Here's how the part is built. I have some questions about the finished solid (model axes, mm). A direction names the side the tool comes from. Coordinates: 2 decimals unless noted, no trailing zeros. Write each loop counter-clockwise with the first axis right and the second up, starting at its lowest first coordinate (ties: lowest second). Pieces come first, ordered by that corner, then holes. Notation, with made-up numbers: (-2.75, 52) -> (26.25, 52) arc R16 cw to (26.25, 76) -> close; hole circle Ø4 at (70.25, 6). An arc over 180 degrees is marked (long way). Put each result on its own line as item: value. Start each with the question number.
Item 1: For pin 1 (2 mm diameter, centred on x = 0, y = 16, fed in from +Z); pin 2 (3 mm diameter, centred on x = -0.5, y = 1, fed in from -Z); pin 3 (1.3 mm diameter, centred on y = -18, z = 5.5, fed in from -X); pin 4 (3 mm diameter, centred on x = -0.5, y = 8, fed in from +Z), each with a flat end and sliding along its axis, tell me the tip position at first contact or that it passes through.
Item 2: I need wall thicknesses on line 1 (Y direction, x = -2.25, z = 6.5); line 2 (Z direction, x = -3.25, y = -4.5); line 3 (Z direction, x = 1.75, y = -3). Which ranges of each line are inside material? Lowest first, please. Write a range as [from, to].
Item 3: I want a section at B-B, the plane x = -1. List the corners of the cut face in (y, z) for me.
Item 4: I want a section at A-A, the plane z = 4.25. List the corners of the cut face in (x, y) for me.
Item 5: I want a section at C-C, the plane y = 16. List the corners of the cut face in (x, z) for me, then the cut area to 3 significant figures.
Item 6: On a 3-axis mill with a long thin cutter (end or side, diameter ignored), from which of +Z, -Z, +X, -X, +Y, -Y can I reach the whole of each face in a straight line? I mean faces 4 (the face through (-2, -17, 7.25)), 5 (the face through (3.43, -23.4, 4.93)), 6 (the face through (-1.4, 1.3, 3)), 7 (the face through (0, 13, 7)). Say none if no direction works.
Item 7: I want a section at D-D, the plane x = 0.75. List the corners of the cut face in (y, z) for me, then the cut area to 3 significant figures.
Item 8: If we mould it in two halves opening along X, with no side actions, what happens to faces 1 (the face through (3, -2, 0)), 2 (the face through (0, -13, 7)), 3 (the face through (0.2, -23.71, 4.93))? For each: released by +X, released by -X, zero draft, split by the parting line, or undercut.
Autodesk Inventor part; units mm, degrees
ref_plane "YZ Plane" through (0, 0, 0) normal (1, 0, 0) x (0, 1, 0)
ref_plane "XZ Plane" through (0, 0, 0) normal (0, 1, 0) x (-1, 0, 0)
ref_plane "XY Plane" through (0, 0, 0) normal (0, 0, 1) x (1, 0, 0)
sketch "Sketch1" plane through (0, 0, 0) normal (0, 0, 1) x (1, 0, 0)
  line L0 (0, -15) -> (0, 15) construction
  line L1 (-4, -15) -> (-4, 15)
  line L2 (4, 15) -> (4, -15)
  arc A0 (-4, -15) -> (0, -19) centre (0, -15) ccw
  arc A1 (4, 15) -> (-4, 15) centre (0, 15) ccw
  line L3 (4, -15) -> (0, -15)
  line L4 (-4, -11) -> (-4, -19)
  line L5 (-4, -19) -> (4, -19)
  line L6 (4, -19) -> (4, -15)
  point P0 (0, 0)
  point P1 (0, 0)
  dimension "d0" = 4
  dimension "d17" = 30
extrude "Extrusion1" add sketch "Sketch1" along normal blind 10 contours L1 A1 L2 L6 L5 A0
sketch "Sketch2" plane through (0, 0, 10) normal (0, 0, 1) x (1, 0, 0)
  line L0 (-4, 15) -> (-4, -15)
  arc A0 (-4, -15) -> (0, -19) centre (0, -15) ccw
  line L1 (4, -19) -> (4, 15)
  arc A1 (4, 15) -> (-4, 15) centre (0, 15) ccw
  circle A2 centre (0, 0) radius 13
  circle A3 centre (0, 0) radius 3.75
  line L2 (0, -19) -> (4, -19)
  dimension "d3" = 26
  dimension "d4" = 7.5
extrude "Extrusion2" cut sketch "Sketch2" against normal blind 7 contours A2 L1 L0 | L0 A2 | A2 L1
sketch "Sketch3" plane through (0, 0, 10) normal (0, 0, 1) x (1, 0, 0)
  circle A0 centre (0, 0) radius 3.75
  circle A1 centre (0, 0) radius 1.75
  line L0 (-4, -12.3693) -> (-4, -15)
  line L1 (4, 12.3693) -> (4, 15)
  arc A2 (4, 12.3693) -> (-4, 12.3693) centre (0, 0) ccw
  arc A3 (4, 15) -> (-4, 15) centre (0, 15) ccw
  arc A4 (-4, -12.3693) -> (4, -12.3693) centre (0, 0) ccw
  arc A5 (-4, -15) -> (0, -19) centre (0, -15) ccw
  line L2 (0, -19) -> (4, -19)
  line L3 (-4, 15) -> (-4, 12.3693)
  line L4 (4, -19) -> (4, -12.3693)
  dimension "d7" = 3.5
extrude "Extrusion3" cut sketch "Sketch3" against normal through all contours A1
sketch "Sketch4" plane through (0, 0, 0) normal (0, 0, -1) x (-1, 0, 0)
  circle A0 centre (0, 0) radius 1.75
  line L0 (4, -15) -> (4, 15)
  arc A1 (4, 15) -> (-4, 15) centre (0, 15) ccw
  line L1 (-4, 15) -> (-4, -19)
  arc A2 (0, -19) -> (4, -15) centre (0, -15) ccw
  circle A3 centre (0, 0) radius 1.75
  line L2 (1.5898, -2.7772) -> (-1.6102, -2.7654)
  line L3 (-1.6102, -2.7654) -> (-3.2, 0.0118)
  line L4 (-3.2, 0.0118) -> (-1.5898, 2.7772)
  line L5 (-1.5898, 2.7772) -> (1.6102, 2.7654)
  line L6 (1.6102, 2.7654) -> (3.2, -0.0118)
  line L7 (3.2, -0.0118) -> (1.5898, -2.7772)
  circle A4 centre (0, 0) radius 3.2
  line L8 (-4, -19) -> (0, -19)
  dimension "d10" = 6.4
extrude "Extrusion4" cut sketch "Sketch4" against normal blind 3 contours L2 L3 L4 L5 L6 L7
sketch "Sketch8" plane through (0, 0, 10) normal (0, 0, 1) x (1, 0, 0)
  arc A0 (4, 12.3693) -> (-4, 12.3693) centre (0, 0) ccw
  line L0 (4, 12.3693) -> (4, 15)
  arc A1 (4, 15) -> (-4, 15) centre (0, 15) ccw
  line L1 (-4, 15) -> (-4, 12.3693)
  circle A2 centre (0, 16) radius 1.75
  dimension "d28" = 3.5
  dimension "d40" = 1
  dimension "d41" = 5.402
extrude "Extrusion8" cut sketch "Sketch8" against normal through all contours A2
sketch "Sketch10" plane through (0, 0, 10) normal (0, 0, 1) x (1, 0, 0)
  circle A0 centre (0, 0) radius 1.75
  circle A1 centre (0, 0) radius 1.75
  circle A2 centre (0, 0) radius 3.75
extrude "Extrusion10" cut sketch "Sketch10" against normal blind 3
sketch "Sketch12" plane through (0, 0, 10) normal (0, 0, 1) x (1, 0, 0)
  arc A0 (-4, -12.3693) -> (4, -12.3693) centre (0, 0) ccw
  line L0 (-4, -12.3693) -> (-4, -15)
  arc A1 (-4, -15) -> (0, -19) centre (0, -15) ccw
  line L1 (0, -19) -> (4, -19)
  line L2 (4, -19) -> (4, -12.3693)
  line L3 (4, -19) -> (4, -24)
  line L4 (4, -24) -> (0, -24)
  line L5 (0, -24) -> (-3.5832, -16.7778)
  arc A2 (-4, -15) -> (0, -19) centre (0, -15) ccw
  arc A3 (-4, -15) -> (0, -19) centre (0, -15) ccw
  line L6 (0, -19) -> (4, -19)
  dimension "d42" = 5
extrude "Extrusion11" add sketch "Sketch12" against normal up to surface (10 mm away) from surface at 0 contours L3 L4 L5 A1 L1
sketch "Sketch9" plane through (-4, -15, 0) normal (-1, 0, 0) x (0, 0, 1)
  line L0 (0, 0) -> (10, 0)
  line L1 (5, -1.5) -> (5, -2.5) construction
  line L2 (2.75, -1.5) -> (2.75, -2.5)
  line L3 (7.25, -2.5) -> (7.25, -1.5)
  arc A0 (7.25, -1.5) -> (2.75, -1.5) centre (5, -1.5) ccw
  arc A1 (2.75, -2.5) -> (7.25, -2.5) centre (5, -2.5) ccw
  line L4 (3, 2.6307) -> (3, 27.3693)
  point P0 (0, 15)
  point P1 (5, -2)
  dimension "d31" = 4.5
  dimension "d34" = 2
  dimension "d45" = 2
extrude "Extrusion9" cut sketch "Sketch9" against normal blind 4
fillet "Fillet4" radius 2 2 edges at (0, -24, 5) (4, -24, 5)
properties part number "rodamiento0.2"
Calculated:
1. pin 1: passes through
1. pin 2: stops at z = 3
1. pin 3: stops at x = 0
1. pin 4: stops at z = 3
2. line 1: y = [-19.46, -19.18], [-14.82, -12.8], [-3, 3], [12.8, 18.31]
2. line 2: z = [0, 3]
2. line 3: z = [0, 7]
3. outline: (-21.98, 0) -> (-2.78, 0) -> (-2.78, 3) -> (-1.44, 3) -> (-1.44, 7) -> (-3.61, 7) -> (-3.61, 3) -> (-12.96, 3) -> (-12.96, 10) -> (-21.98, 10) -> close; (1.44, 3) -> (2.77, 3) -> (2.77, 0) -> (14.56, 0) -> (14.56, 10) -> (12.96, 10) -> (12.96, 3) -> (3.61, 3) -> (3.61, 7) -> (1.44, 7) -> close; (17.44, 0) -> (18.87, 0) -> (18.87, 10) -> (17.44, 10) -> close; hole (-17.5, 2.75) -> (-16.5, 2.75) arc R2.25 ccw to (-16.5, 7.25) -> (-17.5, 7.25) arc R2.25 ccw to start
4. outline: (-4, -14.38) -> (0, -14.38) -> (0, -19.62) -> (-2.17, -19.62) -> (-0.55, -22.89) arc R2 ccw to (1.24, -24) -> (2, -24) arc R2 ccw to (4, -22) -> (4, -12.37) arc R13 cw to (-4, -12.37) -> close; (-4, 12.37) arc R13 cw to (4, 12.37) -> (4, 15) arc R4 ccw to (-4, 15) -> close; circle Ø7.5 at (0, 0); hole circle Ø3.5 at (0, 0); hole circle Ø3.5 at (0, 16)
5. outline: (-3.87, 0) -> (-1.75, 0) -> (-1.75, 10) -> (-3.87, 10) -> close; (1.75, 0) -> (3.87, 0) -> (3.87, 10) -> (1.75, 10) -> close
5. area: 42.5 mm2
6. face 4: -X
6. face 5: +Z, -Z, +X, -Y
6. face 6: -Z
6. face 7: +Z
7. outline: (-23.94, 0) -> (-2.77, 0) -> (-2.77, 3) -> (-1.58, 3) -> (-1.58, 7) -> (-3.67, 7) -> (-3.67, 3) -> (-12.98, 3) -> (-12.98, 10) -> (-23.94, 10) -> close; (1.58, 3) -> (2.77, 3) -> (2.77, 0) -> (14.42, 0) -> (14.42, 10) -> (12.98, 10) -> (12.98, 3) -> (3.67, 3) -> (3.67, 7) -> (1.58, 7) -> close; (17.58, 0) -> (18.93, 0) -> (18.93, 10) -> (17.58, 10) -> close
7. area: 215 mm2
8. face 1: zero draft
8. face 2: undercut
8. face 3: released by -X
